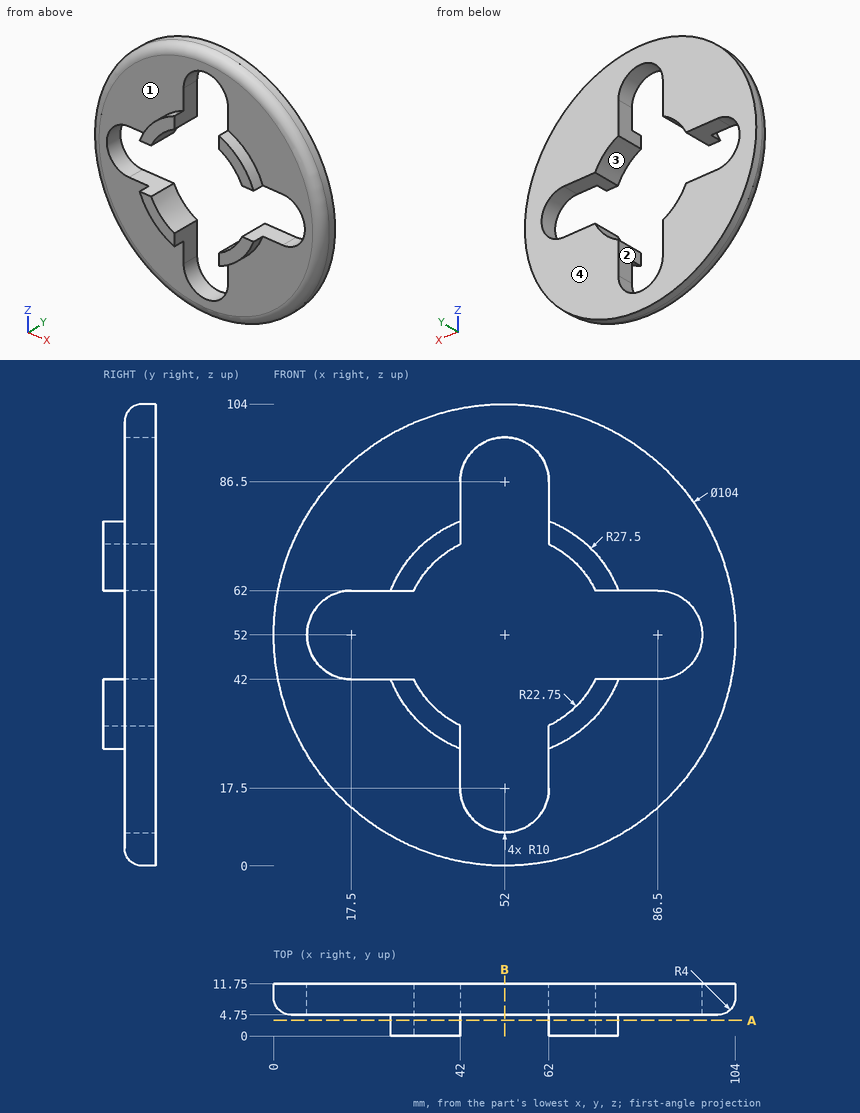
Could you check a few things on this drawing? It's one solid part, dimensions in mm from its lowest x, y, z. A direction names the side the tool comes from. Round coordinates to 2 decimals unless told otherwise and drop trailing zeros. Write each loop counter-clockwise with the first axis right and the second up, starting at its lowest first coordinate (ties: lowest second). Pieces come first, ordered by that corner, then holes. Notation, with made-up numbers: (50.5, 84.5) -> (83.5, 84.5) arc R17 cw to (83.5, 95.5) -> close; hole circle Ø4 at (85, 78.25). An arc over 180 degrees is marked (long way). One line per question, with ' | ' between items. Start each with the question number.
1) On a 3-axis mill with a long thin cutter (end or side, diameter ignored), from which of +Z, -Z, +X, -X, +Y, -Y can I reach the whole of each face in a straight line? I mean the marked faces 3 and 4. Say none if no direction works.
2) Suppose I cut it at B-B on x = 52. Write out the boundary of the cut face in (y, z), then the cut area to 3 significant figures.
3) If we mould it in two halves opening along X, with no side actions, what happens to the marked faces 1 and 2? For each: released by +X, released by -X, zero draft, split by the parting line, or undercut.
4) I'm going to push flat-ended pins straight in: P1, Ø6, axis at y = 4.5, z = 22, coming from the +X side; P2, Ø3, axis at y = 10, z = 46.5, coming from the +X side; P3, Ø3.5, axis at y = 6, z = 80, coming from the -X side. Where does each tip first touch, or does it pass through?
5) Suppose I cut it at A-A on y = 3.5. Write out the boundary of the cut face in (x, z), then the cut area to 3 significant figures.
6) I need wall thicknesses on line 1 (X direction, y = 8.25, z = 89); line 2 (Z direction, x = 36.5, y = 3); line 3 (Y direction, x = 9, z = 66). Which ranges of each line are inside material? Lowest first, please. Write a range as [from, to].
Return value:
1) face 3: +Y, -Y | face 4: +Z, -Z, +X, -X, +Y
2) outline: (4.75, 4) arc R4 ccw to (8.75, 0) -> (11.75, 0) -> (11.75, 7.5) -> (4.75, 7.5) -> close; (4.75, 96.5) -> (11.75, 96.5) -> (11.75, 104) -> (8.75, 104) arc R4 ccw to (4.75, 100) -> close | area: 98.1 mm2
3) face 1: zero draft | face 2: undercut
4) P1: stops at x = 95.17 | P2: stops at x = 103.85 | P3: stops at x = 7.76
5) outline: (26.38, 42) arc R27.5 ccw to (42, 26.38) -> (42, 31.57) arc R22.75 cw to (31.57, 42) -> close; (26.38, 62) -> (31.57, 62) arc R22.75 cw to (42, 72.43) -> (42, 77.62) arc R27.5 ccw to start; (62, 26.38) arc R27.5 ccw to (77.62, 42) -> (72.43, 42) arc R22.75 cw to (62, 31.57) -> close; (62, 72.43) arc R22.75 cw to (72.43, 62) -> (77.62, 62) arc R27.5 ccw to (62, 77.62) -> close | area: 359 mm2
6) line 1: x = [15.51, 42.32], [61.68, 88.49] | line 2: z = [29.28, 35.35], [68.65, 74.72] | line 3: y = [4.75, 11.75]
